For this review, use the dimensioned drawing (mm, ordinates from the lowest corner) and the shaded views. Give positions to 0.01 mm unless a question says otherwise; leave off trailing zeros. Loops run counter-clockwise (first coordinate to the right, second up) from the corner with the lowest first, then second, coordinate; pieces in that order, holes last. Notation, with made-up numbers: M 77,72.5 L 82,72.5 A22 ccw 82,90.5 Z; hole C 82,39.5 d3. An arc over 180 degrees is marked long. Return JSON: item names as keys, results as strings.
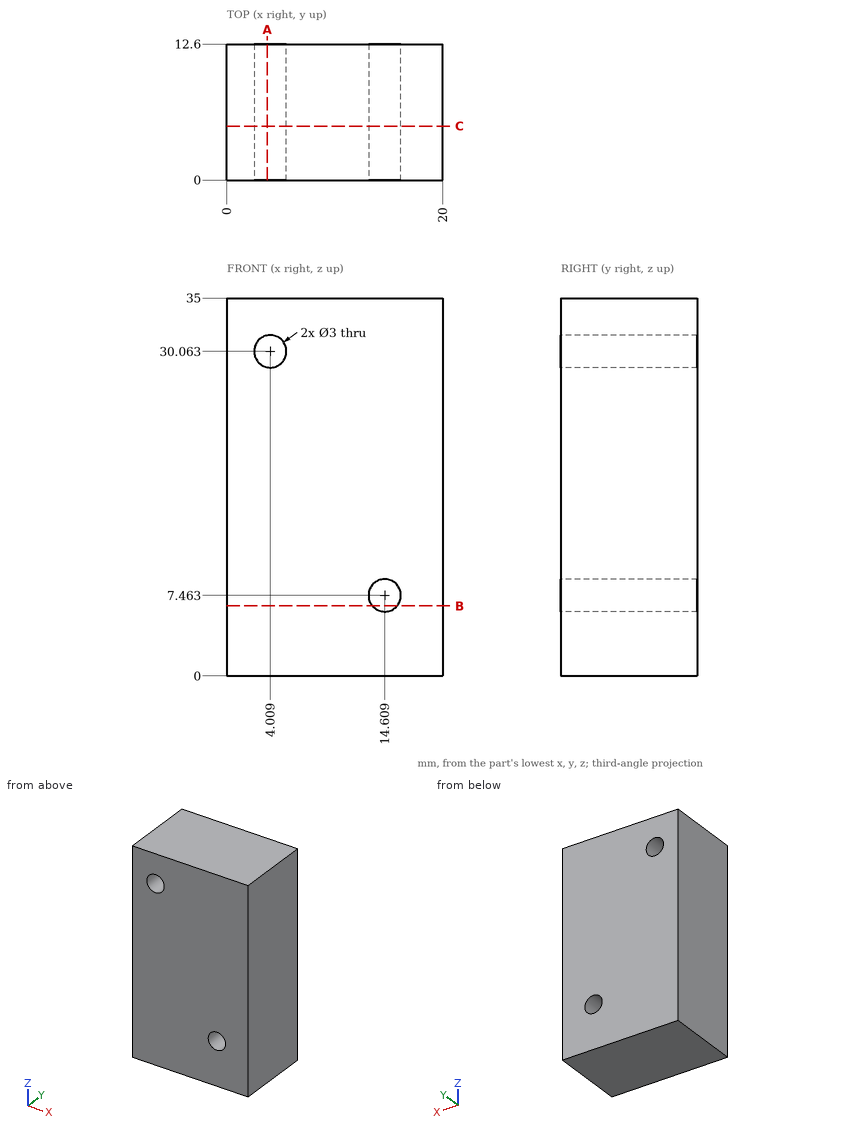
1) Consider section C-C on y = 5. Write out the cut boundary in (x, z).
From the geometry:
{"outline": "M 0,0 L 20,0 L 20,35 L 0,35 Z; hole C 4.01,30.06 d3; hole C 14.61,7.46 d3"}
2) Insertion check: pin 1 (1.8 mm diameter, centred on x = 4.01, z = 30.06, fed in from +Y) (3 decimals). The pin has a flat end and moves straight along its axis. Give the tip position at first contact, or say it passes through.
From the geometry:
{"pin 1": "through"}
3) Wall thickness on L1, parallel to Z at x = 13.25, y = 2.25 (1 decimal); L2, parallel to X at y = 7, z = 31; L3, parallel to Z at x = 15.75, y = 2.75: over which ranges is each line inside the solid? List them lowest first. Write a range as from..to.
From the geometry:
{"L1": "0..6.8, 8.1..35", "L2": "0..2.84, 5.18..20", "L3": "0..6.49, 8.44..35"}
4) Consider section A-A on x = 3.75. Write out the cut boundary in (y, z).
From the geometry:
{"outline": "M 0,0 L 12.6,0 L 12.6,28.59 L 0,28.59 Z; M 0,31.54 L 12.6,31.54 L 12.6,35 L 0,35 Z"}
5) Consider section B-B on z = 6.5. Write out the cut boundary in (x, y).
From the geometry:
{"outline": "M 0,0 L 13.46,0 L 13.46,12.6 L 0,12.6 Z; M 15.76,0 L 20,0 L 20,12.6 L 15.76,12.6 Z"}
